from build123d import *

# Parameters (mm, degrees)
BOSS_EXTRUDE1_DEPTH = 2.54
CUT_EXTRUDE1_REACH  = 129.025
SKETCH2_R           = 1.05
CUT_EXTRUDE2_REACH  = 129.025
SKETCH3_R           = 1.5875


with BuildPart() as part:
    # Sketch1 → Boss-Extrude1 (new body)
    with BuildSketch(Plane(origin=(0, 0, 0), x_dir=(1, 0, 0), z_dir=(0, 1, 0))):
        Polygon((0, 101.6), (76.2, 101.6), (76.2, 78.74), (63.5, 78.74), (63.5, 0), (12.7, 0), (12.7, 78.74), (0, 78.74), align=None)
    extrude(amount=BOSS_EXTRUDE1_DEPTH)

    # Sketch2 → Cut-Extrude1 (cut, up to next)
    with BuildSketch(Plane(origin=(0, 2.54, 0), x_dir=(1, 0, 0), z_dir=(0, 1, 0)), mode=Mode.PRIVATE) as cut_extrude1_sk1:
        with Locations(Location((32.4, 52.6, 0), (0, 0, 270))):
            Circle(SKETCH2_R)
    cut_extrude1_tool1 = extrude(cut_extrude1_sk1.sketch, amount=-CUT_EXTRUDE1_REACH, mode=Mode.PRIVATE) & part.part
    # Sketch2 → Cut-Extrude1 (cut, up to next)
    with BuildSketch(Plane(origin=(0, 2.54, 0), x_dir=(1, 0, 0), z_dir=(0, 1, 0)), mode=Mode.PRIVATE) as cut_extrude1_sk2:
        with Locations(Location((43.8, 52.6, 0), (0, 0, 270))):
            Circle(SKETCH2_R)
    cut_extrude1_tool2 = extrude(cut_extrude1_sk2.sketch, amount=-CUT_EXTRUDE1_REACH, mode=Mode.PRIVATE) & part.part
    # Sketch2 → Cut-Extrude1 (cut, up to next)
    with BuildSketch(Plane(origin=(0, 2.54, 0), x_dir=(1, 0, 0), z_dir=(0, 1, 0)), mode=Mode.PRIVATE) as cut_extrude1_sk3:
        with Locations(Location((43.8, 99.6, 0), (0, 0, 270))):
            Circle(SKETCH2_R)
    cut_extrude1_tool3 = extrude(cut_extrude1_sk3.sketch, amount=-CUT_EXTRUDE1_REACH, mode=Mode.PRIVATE) & part.part
    # Sketch2 → Cut-Extrude1 (cut, up to next)
    with BuildSketch(Plane(origin=(0, 2.54, 0), x_dir=(1, 0, 0), z_dir=(0, 1, 0)), mode=Mode.PRIVATE) as cut_extrude1_sk4:
        with Locations(Location((32.4, 99.6, 0), (0, 0, 270))):
            Circle(SKETCH2_R)
    cut_extrude1_tool4 = extrude(cut_extrude1_sk4.sketch, amount=-CUT_EXTRUDE1_REACH, mode=Mode.PRIVATE) & part.part
    add(cut_extrude1_tool1.solids().sort_by_distance((32.4, 2.54, -52.6))[0], mode=Mode.SUBTRACT)
    add(cut_extrude1_tool2.solids().sort_by_distance((43.8, 2.54, -52.6))[0], mode=Mode.SUBTRACT)
    add(cut_extrude1_tool3.solids().sort_by_distance((43.8, 2.54, -99.6))[0], mode=Mode.SUBTRACT)
    add(cut_extrude1_tool4.solids().sort_by_distance((32.4, 2.54, -99.6))[0], mode=Mode.SUBTRACT)

    # Sketch3 → Cut-Extrude2 (cut, up to next)
    with BuildSketch(Plane(origin=(0, 0, 0), x_dir=(-1, 0, 0), z_dir=(0, -1, 0)), mode=Mode.PRIVATE) as cut_extrude2_sk1:
        with Locations(Location((-23.962149238, 19.05, 0), (0, 0, 90))):
            Circle(SKETCH3_R)
    cut_extrude2_tool1 = extrude(cut_extrude2_sk1.sketch, amount=-CUT_EXTRUDE2_REACH, mode=Mode.PRIVATE) & part.part
    # Sketch3 → Cut-Extrude2 (cut, up to next)
    with BuildSketch(Plane(origin=(0, 0, 0), x_dir=(-1, 0, 0), z_dir=(0, -1, 0)), mode=Mode.PRIVATE) as cut_extrude2_sk2:
        with Locations(Location((-52.237850762, 19.05, 0), (0, 0, 90))):
            Circle(SKETCH3_R)
    cut_extrude2_tool2 = extrude(cut_extrude2_sk2.sketch, amount=-CUT_EXTRUDE2_REACH, mode=Mode.PRIVATE) & part.part
    # Sketch3 → Cut-Extrude2 (cut, up to next)
    with BuildSketch(Plane(origin=(0, 0, 0), x_dir=(-1, 0, 0), z_dir=(0, -1, 0)), mode=Mode.PRIVATE) as cut_extrude2_sk3:
        with Locations(Location((-23.962149238, 90.17, 0), (0, 0, 90))):
            Circle(SKETCH3_R)
    cut_extrude2_tool3 = extrude(cut_extrude2_sk3.sketch, amount=-CUT_EXTRUDE2_REACH, mode=Mode.PRIVATE) & part.part
    # Sketch3 → Cut-Extrude2 (cut, up to next)
    with BuildSketch(Plane(origin=(0, 0, 0), x_dir=(-1, 0, 0), z_dir=(0, -1, 0)), mode=Mode.PRIVATE) as cut_extrude2_sk4:
        with Locations(Location((-52.237850762, 90.17, 0), (0, 0, 90))):
            Circle(SKETCH3_R)
    cut_extrude2_tool4 = extrude(cut_extrude2_sk4.sketch, amount=-CUT_EXTRUDE2_REACH, mode=Mode.PRIVATE) & part.part
    add(cut_extrude2_tool1.solids().sort_by_distance((23.962149, 0, -19.05))[0], mode=Mode.SUBTRACT)
    add(cut_extrude2_tool2.solids().sort_by_distance((52.237851, 0, -19.05))[0], mode=Mode.SUBTRACT)
    add(cut_extrude2_tool3.solids().sort_by_distance((23.962149, 0, -90.17))[0], mode=Mode.SUBTRACT)
    add(cut_extrude2_tool4.solids().sort_by_distance((52.237851, 0, -90.17))[0], mode=Mode.SUBTRACT)


solid = part.part
CAD build for the part. Positions are in the model's coordinates, mm. A direction names the side the tool comes from. Give positions to 0.01 mm unless a question says otherwise; leave off trailing zeros. Write each loop counter-clockwise with the first axis right and the second up, starting at its lowest first coordinate (ties: lowest second). Pieces come first, ordered by that corner, then holes. Notation, with made-up numbers: (84, -23) - (140, -23) arc R18 cw to (140, -16) - close; hole circle Ø1 at (-39.75, 31.25). An arc over 180 degrees is marked (long way). Put each result on its own line as item: value.
(1) Saw through at B-B (x = 32.4). List the corners of the cut face in (y, z), then the cut area to 3 significant figures.
Working result:
outline: (0, -101.6) - (2.54, -101.6) - (2.54, -100.65) - (0, -100.65) - close; (0, -98.55) - (2.54, -98.55) - (2.54, -53.65) - (0, -53.65) - close; (0, -51.55) - (2.54, -51.55) - (2.54, 0) - (0, 0) - close
area: 247 mm^2
(2) Wall check: L1, parallel to X at y = 0.7, z = -90.17; L2, parallel to X at y = 1.7, z = -99.6; L3, parallel to X at y = 2.25, z = -62. Give the ranges that are in metal, low to high.
Working result:
L1: 0 to 22.37, 25.55 to 50.65, 53.83 to 76.2
L2: 0 to 31.35, 33.45 to 42.75, 44.85 to 76.2
L3: 12.7 to 63.5
(3) Drop flat-ended pins along their axis: pin 1 Ø3.5 at (x, z) = (32.4, -99.6) entering from +Y; pin 2 Ø1.3 at (y, z) = (1.5, -52.5) entering from -X; pin 3 Ø1.3 at (x, z) = (43.8, -52.6) entering from +Y; pin 4 Ø0.8 at (x, y) = (6.5, 1) entering from +Z. Give the stop position or say it passes through.
Working result:
pin 1: y = 2.54
pin 2: x = 12.7
pin 3: through
pin 4: z = -78.74
(4) Saw through at D-D (z = -58.5). List the corners of the cut face in (x, y).
Working result:
outline: (12.7, 0) - (63.5, 0) - (63.5, 2.54) - (12.7, 2.54) - close
(5) Tool access for faces 1 (the flat face through (70, 1, -78.74)), 2 (the flat face through (38, 1, 0)), 3 (the flat face through (12.7, 1, -39)): list every direction of +Z, -Z, +X, -X, +Y, -Y with a clear straight run to the whole face (end or side of a thin tool).
Working result:
face 1: +Z, +X, +Y, -Y
face 2: +Z, +X, -X, +Y, -Y
face 3: +Z, -X, +Y, -Y
(6) Pull direction X, two halves, no side cores. Call faces 4 (the cylindrical face through (33.44, 1.29, -52.74)), 5 (the flat face through (39, 0, -52)), 6 (the flat face through (63.5, 1, -40)): released by +X, released by -X, zero draft, split by the parting line, or undercut.
Working result:
face 4: undercut
face 5: zero draft
face 6: released by +X
(7) Saw through at A-A (z = -19.05). List the corners of the cut face in (x, y), then the cut area to 3 significant figures.
Working result:
outline: (12.7, 0) - (22.37, 0) - (22.37, 2.54) - (12.7, 2.54) - close; (25.55, 0) - (50.65, 0) - (50.65, 2.54) - (25.55, 2.54) - close; (53.83, 0) - (63.5, 0) - (63.5, 2.54) - (53.83, 2.54) - close
area: 113 mm^2
(8) Saw through at C-C (y = 1.5). Count the separate pieces of the cut face and the enclosed holes in it, then the cut area to 3 significant figures.
Working result:
separate pieces: 1
enclosed holes: 8
area: 5,700 mm^2
